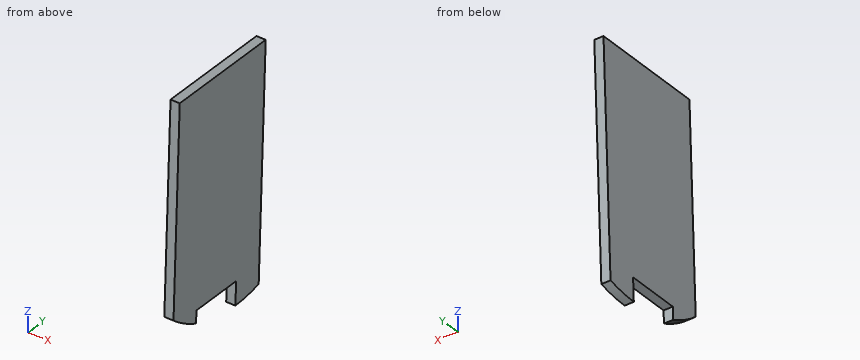
from build123d import *

# Parameters (mm, degrees)
SALIENTE_EXTRUIR2_DEPTH = 5
CROQUIS3_W              = 15
CROQUIS3_H              = 30
CORTAR_EXTRUIR2_DEPTH   = 10


with BuildPart() as part:
    # Croquis2 → Saliente-Extruir2 (new body)
    with BuildSketch(Plane(origin=(2.49030702, 0, -0.073938452), x_dir=(-0.029677418771206387, 0, -0.999559528399924), z_dir=(0.999559528399924, 0, -0.029677418771206387))):
        with BuildLine():
            Line((-0.326611286, 53.303101177), (116.885919238, 53.303101177))
            Line((116.885919238, 53.303101177), (128.299912644, 53.303101177))
            ThreePointArc((128.299912644, 53.303101177), (128.897751071, 19.112162844), (114.059307952, -11.696898823))
            Line((114.059307952, -11.696898823), (-0.326611286, -11.696898823))
            Line((-0.326611286, -11.696898823), (-0.326611286, 53.303101177))
        make_face()
    extrude(amount=-SALIENTE_EXTRUIR2_DEPTH)

    # Croquis3 → Cortar-Extruir2 (cut)
    with BuildSketch(Plane(origin=(2.49030702, 0, -0.073938452), x_dir=(-0.029677418771206443, 0, -0.999559528399924), z_dir=(0.999559528399924, 0, -0.029677418771206443))):
        with Locations((125.186431424, 20.803101177)):
            Rectangle(CROQUIS3_W, CROQUIS3_H)
    extrude(amount=-CORTAR_EXTRUIR2_DEPTH, mode=Mode.SUBTRACT)


solid = part.part
Input: part model. Units: mm. Frame: model coordinates. Give positions to 0.01 mm unless a question says otherwise; leave off trailing zeros. Order: outer loops, then holes, each group sorted by start corner. A loop starts at its lowest first (then second) coordinate and runs counter-clockwise, first axis right, second up. Notation, with made-up numbers: (85, -4.5) -> (139, -4.5) arc R8 cw to (139, 6.5) -> close; hole circle Ø2 at (29, 65.25). An arc over 180 degrees is marked (long way). Use one line per item in the form item = value.
1) First-contact query: pin 1 Ø1 at (y, z) = (26, -40) entering from +X; pin 2 Ø4 at (y, z) = (12, -39.5) entering from +X; pin 3 Ø6 at (y, z) = (18.5, -26) entering from +X. Flat tips, straight axial feed; report the tip coordinate or a pass-through.
Response values:
pin_1 = 1.32
pin_2 = 1.38
pin_3 = 1.81
2) Line query: probe 1 along X at (y, z) = (40.5, -76); probe 2 along X at (y, z) = (50, -104). Output: solid intervals per line, ascending.
Response values:
probe_1 = -4.77 to 0.24
probe_2 = -5.6 to -0.6
3) Section B-B, the plane x = 0.5. Return loops of the section in (y, z), and give its area (3 significant figures).
Response values:
outline = (-11.7, -67.11) -> (53.3, -67.11) -> (53.3, 0.31) -> (-11.7, 0.31) -> close
area = 4,380 mm^2
4) Section A-A, the plane y = 24.5. Return loops of the section in (x, z), and give its area (3 significant figures).
Response values:
outline = (-6, -117.56) -> (-1, -117.71) -> (2.5, 0.25) -> (-2.5, 0.4) -> close
area = 590 mm^2
